The model under review builds one solid part; all positions refer to its coordinate system, in mm. A direction names the side the tool comes from. Coordinates: 2 decimals unless noted, no trailing zeros. Loops run counter-clockwise (first coordinate to the right, second up) from the corner with the lowest first, then second, coordinate; pieces in that order, holes last. Notation, with made-up numbers: (67.5, 45.25) - (104.5, 45.25) arc R13 cw to (104.5, 50.25) - close; hole circle Ø8 at (46, 76). An arc over 180 degrees is marked (long way). One line per item, written item: value. Start each with the question number.
1. We need section A-A, the plane z = -107. Give the boundary of the cut face in (x, y).
2. We need section B-B, the plane x = -79.5. Give the boundary of the cut face in (y, z).
3. Mouldability with a two-part tool opening along X and no side actions: class faces 1 (the face through (-2, 0, -3)), 2 (the face through (90.85, 21, 3)), 3 (the face through (115, 13, 3)) as +X half, -X half, draft (parallel to the pull), parting line (faces both ways), or undercut.
4. Insertion check: P1, Ø3, axis at x = -47.5, z = -51, coming from the -Y side; P2, Ø10.5, axis at x = 80.5, z = 14.5, coming from the +Y side. Each pin has a flat end and moves straight along its axis. Give the tip position at first contact, or say it passes through.
5. To check wall thickness, follow line 1 (X direction, y = 22.5, z = 21); line 2 (Y direction, x = 77, z = 148.5). State the ranges of each line that lie inside material, in increasing order.
6. For faces 4 (the face through (-80, 16, -3)), 5 (the face through (-1, 26, -3)), list the 3-axis set-ups (+Z, -Z, +X, -X, +Y, -Y) from which the entire face can be reached by the end or side of a thin tool; tool diameter is ignored.
from build123d import *

# Parameters (mm, degrees)
SKETCH1_W           = 230
SKETCH1_H           = 420
BOSS_EXTRUDE1_DEPTH = 26
SKETCH2_W           = 21
SKETCH2_H           = 420
CUT_EXTRUDE1_DEPTH  = 10


with BuildPart() as part:
    # Sketch1 → Boss-Extrude1 (new body)
    with BuildSketch(Plane(origin=(0, 0, 0), x_dir=(1, 0, 0), z_dir=(0, 1, 0))):
        Rectangle(SKETCH1_W, SKETCH1_H)
    extrude(amount=BOSS_EXTRUDE1_DEPTH)

    # Sketch2 → Cut-Extrude1 (cut)
    with BuildSketch(Plane(origin=(0, 26, 0), x_dir=(1, 0, 0), z_dir=(0, 1, 0))):
        with Locations((-80.35, 0)):
            Rectangle(SKETCH2_W, SKETCH2_H)
        with Locations((80.35, 0)):
            Rectangle(SKETCH2_W, SKETCH2_H)
    extrude(amount=-CUT_EXTRUDE1_DEPTH, mode=Mode.SUBTRACT)


solid = part.part
Findings below:
1. outline: (-115, 0) - (115, 0) - (115, 26) - (90.85, 26) - (90.85, 16) - (69.85, 16) - (69.85, 26) - (-69.85, 26) - (-69.85, 16) - (-90.85, 16) - (-90.85, 26) - (-115, 26) - close
2. outline: (0, -210) - (16, -210) - (16, 210) - (0, 210) - close
3. face 1: draft
3. face 2: undercut
3. face 3: +X half
4. P1: y = 0
4. P2: y = 16
5. line 1: -115 to -90.85, -69.85 to 69.85, 90.85 to 115
5. line 2: 0 to 16
6. face 4: +Z, -Z, +Y
6. face 5: +Z, -Z, +X, -X, +Y
